Build history of the part. All positions in model axes, mm. A direction names the side the tool comes from. Round coordinates to 2 decimals unless told otherwise and drop trailing zeros. Loops run counter-clockwise (first coordinate to the right, second up) from the corner with the lowest first, then second, coordinate; pieces in that order, holes last. Notation, with made-up numbers: M -16.75,86 L 23.25,86 A22 ccw 23.25,93 Z; hole C 7,-24.5 d6. An arc over 180 degrees is marked long. One line per item, written item: value.
```python
from build123d import *

# Parameters (mm, degrees)
F1_DEPTH = 3
F3_DEPTH = 25
F4_W     = 5
F4_H     = 15
F4_W_2   = 10
F4_H_2   = 4
F5_DEPTH = 10


with BuildPart() as f1:
    # F0 (on Front) → F1 (new body)
    with BuildSketch(Plane.XZ):
        Polygon((70, 45), (-70, 45), (-70, 7.5), (-90, 7.5), (-90, -7.5), (-70, -7.5), (-70, -45), (70, -45), (70, -7.5), (90, -7.5), (90, 7.5), (70, 7.5), align=None)
    extrude(amount=F1_DEPTH)

    # F2 (on face) → F3 (cut)
    with BuildSketch(Plane.XZ.offset(3)):
        Polygon((-28, 37), (-60.8, 37), (-60.8, 3), (-74.339576, 3), (-74.339576, -3), (-60.8, -3), (-60.8, -37), (-28, -37), (-28, -3), (-48, -3), (-48, 3), (-28, 3), align=None)
        Polygon((0, 37), (-22, 37), (-22, 3), (-3, 3), (-3, 13), (0, 13), (3, 13), (3, 3), (22, 3), (22, 37), align=None)
        Polygon((-3, -13), (-3, -3), (-22, -3), (-22, -37), (0, -37), (22, -37), (22, -3), (3, -3), (3, -13), (0, -13), align=None)
        Polygon((60.8, 3), (60.8, 37), (28, 37), (28, 3), (48, 3), (48, -3), (28, -3), (28, -37), (60.8, -37), (60.8, -3), (74.339576, -3), (74.339576, 3), align=None)
    extrude(amount=-F3_DEPTH, mode=Mode.SUBTRACT)

    # F4 (on face) → F5 (join)
    with BuildSketch(Plane.XZ.offset(3)):
        with Locations((-87.5, 0)):
            Rectangle(F4_W, F4_H)
        with Locations((87.5, 0)):
            Rectangle(F4_W, F4_H)
        with Locations((-32.5, 43)):
            Rectangle(F4_W_2, F4_H_2)
        with Locations((32.5, 43)):
            Rectangle(F4_W_2, F4_H_2)
    extrude(amount=F5_DEPTH)


solid = f1.part
```
Item 1: Slice it at A-A, the plane z = -23.5. Give the cut face in (x, y).
Check values:
outline: M -70,-3 L -60.8,-3 L -60.8,0 L -70,0 Z; M -28,-3 L -22,-3 L -22,0 L -28,0 Z; M 22,-3 L 28,-3 L 28,0 L 22,0 Z; M 60.8,-3 L 70,-3 L 70,0 L 60.8,0 Z
Item 2: Slice it at D-D, the plane z = 9.5. Give the cut face in (x, y), and give its area (3 significant figures).
Check values:
outline: M -70,-3 L -60.8,-3 L -60.8,0 L -70,0 Z; M -28,-3 L -22,-3 L -22,0 L -28,0 Z; M -3,-3 L 3,-3 L 3,0 L -3,0 Z; M 22,-3 L 28,-3 L 28,0 L 22,0 Z; M 60.8,-3 L 70,-3 L 70,0 L 60.8,0 Z
area: 109 mm2
Item 3: Slice it at C-C, the plane y = -7.75. Give the cut face in (x, z).
Check values:
outline: M -90,-7.5 L -85,-7.5 L -85,7.5 L -90,7.5 Z; M -37.5,41 L -27.5,41 L -27.5,45 L -37.5,45 Z; M 27.5,41 L 37.5,41 L 37.5,45 L 27.5,45 Z; M 85,-7.5 L 90,-7.5 L 90,7.5 L 85,7.5 Z
Item 4: Pull direction X, two halves, no side cores. Call faces 5 (the face through (-37.5, -8, 43)), 6 (the face through (90, -6, 0)), 7 (the face through (-85, -8, 0)), 8 (the face through (32, -8, 41)): pulls with the +X half, pulls with the -X half, needs draft (parallel to the pull), parting line crosses it, or undercut.
Check values:
face 5: pulls with the -X half
face 6: pulls with the +X half
face 7: undercut
face 8: needs draft
Item 5: Wall check: line 1 along X through (y, z) = (-0.75, 24); line 2 along X through (y, z) = (-1, -6); line 3 along X through (y, z) = (-1.25, 12.5). Give the ranges that are in metal, low to high.
Check values:
line 1: x = -70 to -60.8, -28 to -22, 22 to 28, 60.8 to 70
line 2: x = -90 to -60.8, -28 to -22, -3 to 3, 22 to 28, 60.8 to 90
line 3: x = -70 to -60.8, -28 to -22, -3 to 3, 22 to 28, 60.8 to 70
Item 6: Which spindle directions (+Z, -Z, +X, -X, +Y, -Y) get a long thin tool onto all of the face, cutting with end or side? Do faces 1 (the face through (85, -2, 7.5)), 2 (the face through (-33, -8, 41)), 3 (the face through (84, -2, -7.5)), 4 (the face through (-27.5, -8, 43)). Say none if no direction does.
Check values:
face 1: +Z, +X, +Y, -Y
face 2: -Z, +X, -X, -Y
face 3: -Z, +X, +Y, -Y
face 4: +Z, -Z, -Y
Item 7: Slice it at B-B, the plane x = -7. Give the cut face in (y, z), and give its area (3 significant figures).
Check values:
outline: M -3,-45 L 0,-45 L 0,-37 L -3,-37 Z; M -3,-3 L 0,-3 L 0,3 L -3,3 Z; M -3,37 L 0,37 L 0,45 L -3,45 Z
area: 66.0 mm2
Item 8: Drop flat-ended pins along their axis: P1, Ø3.5, axis at y = -1, z = -31, coming from the -X side; P2, Ø2, axis at y = -3, z = 33, coming from the +X side; P3, Ø10, axis at x = -48, z = 34, coming from the -Y side. Give the stop position or say it passes through.
Check values:
P1: stops at x = -70
P2: stops at x = 70
P3: stops at y = -3
